Solid Edge part; units mm, degrees
sketch "Sketch1" plane through (0, 0, 0) normal (0, 0, 1) x (1, 0, 0)
  circle A0 centre (0, 0) radius 5.2197
extrude "Protrusion1" add sketch "Sketch1" along normal blind 3.2258
sketch "Sketch2" plane through (0, 0, 0) normal (0, 0, -1) x (1, 0, 0)
  circle A0 centre (0, 0) radius 2.413
extrude "Protrusion2" add sketch "Sketch2" along normal blind 15.8242
sketch "Sketch3" plane through (0, 0, -15.8242) normal (0, 0, -1) x (1, 0, 0)
  circle A0 centre (0, 0) radius 2.4127
extrude "Cutout1" cut sketch "Sketch3" against normal blind 15.8084 flip side to cut
chamfer "Chamfer_1" distance 0.3619 angle 45 1 edges at (-2.4127, 0, -15.8242)
sketch "Sketch4" plane through (0, 0, 3.2258) normal (0, 0, 1) x (1, 0, 0)
  line L0 (-0.9165, 1.5875) -> (0.9165, 1.5875)
  line L1 (1.8331, 0) -> (0.9165, 1.5875)
  line L2 (0.9165, -1.5875) -> (1.8331, 0)
  line L3 (-0.9165, -1.5875) -> (0.9165, -1.5875)
  line L4 (-1.8331, 0) -> (-0.9165, -1.5875)
  line L5 (-0.9165, 1.5875) -> (-1.8331, 0)
extrude "Cutout2" cut sketch "Sketch4" against normal blind 2.1505
sketch "Sketch5" plane through (0, 0, 0) normal (0, -1, 0) x (1, 0, 0)
  line L0 (5.2197, 3.2258) -> (2.4156, 0)
  line L1 (2.4156, 0) -> (5.2197, 0)
  line L2 (5.2197, 0) -> (5.2197, 3.2258)
revolve "RevolvedCutout1" cut sketch "Sketch5" angle 360 about axis through (0, 0, 14.0017) along (0, 0, -1)
properties part number "24101615"
Here's how the part is built. I have some questions about the finished solid (model axes, mm). A direction names the side the tool comes from. Round coordinates to 2 decimals unless told otherwise and drop trailing zeros. Order: outer loops, then holes, each group sorted by start corner. A loop starts at its lowest first (then second) coordinate and runs counter-clockwise, first axis right, second up. Notation, with made-up numbers: (83, 73) -> (95, 73) arc R26 cw to (95, 108) -> close; hole circle Ø6 at (89.5, 59.25). An arc over 180 degrees is marked (long way). Use a Markdown table: item, result. Add a question column.
(1) For faces 1 (the face through (0, -2, 3.226)), 2 (the face through (-1.381, -0.783, 2.166)), which set-ups out of +Z, -Z, +X, -X, +Y, -Y let a thin tool reach every point of the face, with its end or its side?
(2) If we mould it in two halves opening along X, with no side actions, what happens to faces 3 (the face through (-0.314, -2.392, -7.847)), 4 (the face through (0, 0, -15.824)), 5 (the face through (-1.37, 0.8, 2.17))? For each: released by +X, released by -X, zero draft, split by the parting line, or undercut.
(3) For pin 1 Ø5 at (x, z) = (-0.5, -14) entering from -Y; pin 2 Ø2 at (x, z) = (0, 2) entering from -Y; pin 3 Ø1.5 at (y, z) = (-2.5, -12.5) entering from +X, each with a flat end and sliding along its axis, tell me the tip position at first contact or that it passes through.
(4) Suppose I cut it at B-B, the plane z = -14.5. Please give me the cut outline in (x, y).
(5) I need wall thicknesses on line 1 along Z through (x, y) = (1.75, 1.5); line 2 along Z through (x, y) = (-1, 4.25); line 3 along X through (y, z) = (-2, -9). Which ranges of each line are inside material? Lowest first, please.
Verdict:
| question | item | result |
|---|---|---|
| 1 | face 1 | +Z, +X, -X, +Y, -Y |
| 1 | face 2 | +Z |
| 2 | face 3 | split by the parting line |
| 2 | face 4 | zero draft |
| 2 | face 5 | undercut |
| 3 | pin 1 | y = -2.41 |
| 3 | pin 2 | y = -5.02 |
| 3 | pin 3 | x = 1.66 |
| 4 | outline | circle Ø4.83 at (0, 0) |
| 5 | line 1 | -15.57 to 3.23 |
| 5 | line 2 | 2.24 to 3.23 |
| 5 | line 3 | -1.35 to 1.35 |
